The model under review builds one solid part; all positions refer to its coordinate system, in mm. Face numbers are marked on the shaded views. Give positions to 0.01 mm unless a question says otherwise; leave off trailing zeros. Loops run counter-clockwise (first coordinate to the right, second up) from the corner with the lowest first, then second, coordinate; pieces in that order, holes last. Notation, with made-up numbers: M 27.5,-15 L 65.5,-15 A8 ccw 65.5,-7 Z; hole C -17,88 d10. An arc over 180 degrees is marked long. Return JSON: item names as keys, results as strings.
```python
from build123d import *

# Parameters (mm, degrees)
SKETCH1_R           = 3
BOSS_EXTRUDE1_DEPTH = 2.6
FILLET1_R           = 0.1
SKETCH3_R           = 2.9
BOSS_EXTRUDE2_DEPTH = 0.1
SKETCH2_R           = 0.5
CUT_EXTRUDE1_DEPTH  = 1
SKETCH4_R           = 0.3
BOSS_EXTRUDE3_DEPTH = 2.8
CHAMFER1_SIZE       = 0.05


with BuildPart() as part:
    # Sketch1 → Boss-Extrude1 (new body)
    with BuildSketch(Plane(origin=(0, 0, 0), x_dir=(1, 0, 0), z_dir=(0, 1, 0))):
        with Locations(Location((0, 0, 0), (0, 0, 270))):
            Circle(SKETCH1_R)
    extrude(amount=BOSS_EXTRUDE1_DEPTH)

    # Fillet1
    fillet1_edges = [part.edges().sort_by_distance(p)[0] for p in [
        (0, 0, -3),
        (0, 2.6, -3),
    ]]
    fillet(fillet1_edges, radius=FILLET1_R)

    # Sketch3 → Boss-Extrude2 (add)
    with BuildSketch(Plane(origin=(0, 2.6, 0), x_dir=(1, 0, 0), z_dir=(0, 1, 0))):
        with Locations(Location((0, 0, 0), (0, 0, 270))):
            Circle(SKETCH3_R)
    extrude(amount=BOSS_EXTRUDE2_DEPTH)

    # Sketch2 → Cut-Extrude1 (cut)
    with BuildSketch(Plane(origin=(0, 2.7, 0), x_dir=(1, 0, 0), z_dir=(0, 1, 0))):
        with Locations(Location((0, 0, 0), (0, 0, 270))):
            Circle(SKETCH2_R)
    extrude(amount=-CUT_EXTRUDE1_DEPTH, mode=Mode.SUBTRACT)

    # Sketch4 → Boss-Extrude3 (add)
    with BuildSketch(Plane.XZ):
        with Locations(Location((-0.95, 1, 0), (0, 0, 90))):
            Circle(SKETCH4_R)
        with Locations(Location((0.95, 1, 0), (0, 0, 90))):
            Circle(SKETCH4_R)
    extrude(amount=BOSS_EXTRUDE3_DEPTH)

    # Chamfer1
    chamfer1_edges = [part.edges().sort_by_distance(p)[0] for p in [
        (-0.95, -2.8, 0.7),
        (0.95, -2.8, 0.7),
    ]]
    chamfer(chamfer1_edges, length=CHAMFER1_SIZE)


solid = part.part
```
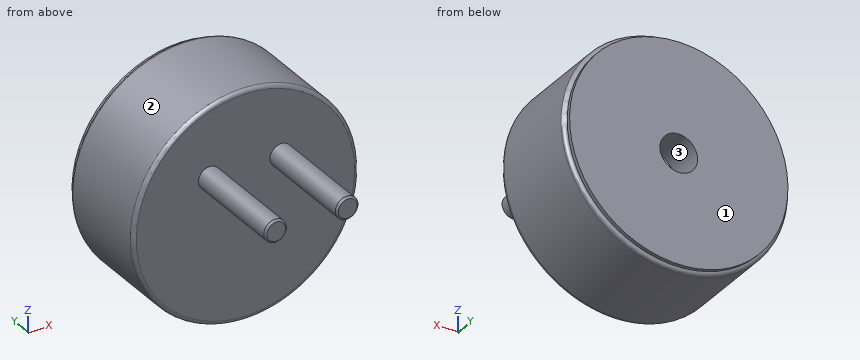
1) Insertion check: pin 1 (0.5 mm diameter, centred on x = 0, z = 0, fed in from +Y). The pin has a flat end and moves straight along its axis. Give the tip position at first contact, or say it passes through.
From the geometry:
{"pin 1": "y = 1.7"}
2) Wall thickness on L1, parallel to X at y = 2.05, z = 0; L2, parallel to Y at x = 0.25, z = -1.75; L3, parallel to X at y = 0.85, z = -2: over which ranges is each line inside the solid? List them lowest first. Write a range as from..to.
From the geometry:
{"L1": "-3..-0.5, 0.5..3", "L2": "0..2.7", "L3": "-2.24..2.24"}
3) Consider section A-A on x = 0. Write out the cut boundary in (y, z).
From the geometry:
{"outline": "M 0,-2.9 A0.1 ccw 0.1,-3 L 2.5,-3 A0.1 ccw 2.6,-2.9 L 2.7,-2.9 L 2.7,-0.5 L 1.7,-0.5 L 1.7,0.5 L 2.7,0.5 L 2.7,2.9 L 2.6,2.9 A0.1 ccw 2.5,3 L 0.1,3 A0.1 ccw 0,2.9 Z"}
4) The part is to be moulded in two halves that separate along X. For the marked faces 1, 2 and 3, say which applies: released by +X, released by -X, zero draft, split by the parting line, or undercut.
From the geometry:
{"face 1": "zero draft", "face 2": "split by the parting line", "face 3": "undercut"}
5) Consider section D-D on y = -1.3. Write out the cut boundary in (x, z).
From the geometry:
{"outline": "C -0.95,1 d0.6; C 0.95,1 d0.6"}
6) Consider section B-B on z = 0. Write out the cut boundary in (x, y), then the cut area to 3 significant figures.
From the geometry:
{"outline": "M -3,0.1 A0.1 ccw -2.9,0 L 2.9,0 A0.1 ccw 3,0.1 L 3,2.5 A0.1 ccw 2.9,2.6 L 2.9,2.7 L 0.5,2.7 L 0.5,1.7 L -0.5,1.7 L -0.5,2.7 L -2.9,2.7 L -2.9,2.6 A0.1 ccw -3,2.5 Z", "area": "15.2 mm²"}
7) Consider section C-C on y = 2.25. Write out the cut boundary in (x, z).
From the geometry:
{"outline": "C 0,0 d6; hole C 0,0 d1"}
